from build123d import *

# Parameters (mm, degrees)
PAD_DEPTH       = 85
PAD001_DEPTH    = 6
POCKET_DEPTH    = 42.401
POCKET001_DEPTH = 48.001
FILLET_R        = 1
CHAMFER_SIZE    = 1


with BuildPart() as part:
    # Sketch → Pad (new body)
    with BuildSketch(Plane.XY):
        with BuildLine():
            Line((40, 30), (40, 0))
            ThreePointArc((0, -40), (28.284271, -28.284271), (40, 0))
            Line((0, -40), (0, -42.4))
            ThreePointArc((0, -42.4), (29.981328, -29.981328), (42.4, 0))
            Line((42.4, 48), (42.4, 0))
            Line((0, 48), (42.4, 48))
            Line((0, 48), (0, 40))
            Line((0, 40), (30, 40))
            ThreePointArc((40, 30), (37.071068, 37.071068), (30, 40))
        make_face()
    pad = extrude(amount=PAD_DEPTH)

    # Mirrored: Pad across Sketch V_Axis
    add(pad.mirror(Plane(origin=(0, 0, 0), x_dir=(0, 0, 1), z_dir=(1, 0, 0))))

    # Sketch001 → Pad001 (join)
    with BuildSketch(Plane.XY):
        Polygon((6, -41.507187), (6, -6), (40.95602, -6), (40.95602, 6), (6, 6), (6, 41.507187), (-6, 41.507187), (-6, 6), (-40.95602, 6), (-40.95602, -6), (-6, -6), (-6, -41.507187), align=None)
    extrude(amount=PAD001_DEPTH)

    # Sketch002 → Pocket (cut, through all)
    with BuildSketch(Plane.XZ):
        with BuildLine():
            Line((0, 53.283252), (-12.698919, 35.147317))
            ThreePointArc((-12.698919, 35.147317), (-13.7168, 19.617441), (-0.411638, 11.54367))
            Line((-0.411638, 11.54367), (0.411638, 11.54367))
            ThreePointArc((0.411638, 11.54367), (13.7168, 19.617441), (12.698919, 35.147317))
            Line((12.698919, 35.147317), (0, 53.283252))
        make_face()
    extrude(amount=POCKET_DEPTH, mode=Mode.SUBTRACT)

    # Sketch003 → Pocket001 (cut, through all)
    with BuildSketch(Plane.XZ):
        with BuildLine():
            ThreePointArc((27.5, 65.454356), (30, 54), (32.5, 65.454356))
            Line((32.5, 65.454356), (32.5, 75))
            ThreePointArc((32.5, 75), (30, 77.5), (27.5, 75))
            Line((27.5, 75), (27.5, 65.454356))
        make_face()
        with BuildLine():
            ThreePointArc((-32.5, 65.454356), (-30, 54), (-27.5, 65.454356))
            Line((-27.5, 65.454356), (-27.5, 75))
            ThreePointArc((-27.5, 75), (-30, 77.5), (-32.5, 75))
            Line((-32.5, 75), (-32.5, 65.454356))
        make_face()
        with BuildLine():
            ThreePointArc((-2.5, 18.617909), (0, 7.163552), (2.5, 18.617909))
            Line((2.5, 18.617909), (2.5, 28.163552))
            ThreePointArc((2.5, 28.163552), (0, 30.663552), (-2.5, 28.163552))
            Line((-2.5, 28.163552), (-2.5, 18.617909))
        make_face()
    extrude(amount=-POCKET001_DEPTH, mode=Mode.SUBTRACT)

    # Fillet
    fillet_edges = [part.edges().sort_by_distance(p)[0] for p in [
        (-40, 15, 85),
        (-28.284271, -28.284271, 85),
        (0, -41.2, 85),
        (-29.981328, -29.981328, 85),
        (-42.4, 24, 85),
        (-21.2, 48, 85),
        (0, 44, 85),
        (-15, 40, 85),
        (-37.071068, 37.071068, 85),
    ]]
    fillet(fillet_edges, radius=FILLET_R)

    # Chamfer
    chamfer_edges = [part.edges().sort_by_distance(p)[0] for p in [
        (-6, 23, 6),
        (-23, 6, 6),
        (-22.77372, -6, 6),
        (-6, -22.77372, 6),
        (6, -22.77372, 6),
        (22.77372, -6, 6),
        (23, 6, 6),
        (6, 23, 6),
    ]]
    chamfer(chamfer_edges, length=CHAMFER_SIZE)


solid = part.part
Geometry: final body of the model. Coordinates: model frame, mm. A direction names the side the tool comes from. Coordinates: 2 decimals unless noted, no trailing zeros. Order: outer loops, then holes, each group sorted by start corner. A loop starts at its lowest first (then second) coordinate and runs counter-clockwise, first axis right, second up.
(1) Section query A-A (z = 60). Return the cut outline in (x, y).
(2) Draft query along Y for faces 5 (the face through (27.5, 44, 70)), 6 (the face through (23, -6, 2)). Return one class per face: pulls with the +Y half, pulls with the -Y half, needs draft (parallel to the pull), parting line crosses it, or undercut.
(3) Section query D-D (z = 26). Return the cut outline in (x, y).
(4) Material intervals for probe 1 along X at (y, z) = (41.25, 60); probe 2 along X at (y, z) = (30, 76); probe 3 along Z at (x, y) = (0, 42), sorted ascending.
(5) First-contact query: pin 1 (7 mm diameter, centred on x = 30, z = 60, fed in from +Y); pin 2 (4 mm diameter, centred on y = -32, z = 68, fed in from +X); pin 3 (5.5 mm diameter, centred on x = -17, z = 2, fed in from -Y). Flat tips, straight axial feed; report the tip coordinate or a pass-through.
(6) Section query C-C (y = 33.5). State how many separate pieces and enclosed holes the cut face has, plus the area to 3 significant figures.
(7) Section query B-B (z = 45.5). Return the cut outline in (x, y), plus the area to 3 significant figures.
(8) Access query for faces 1 (the face through (13.6, -39, 19.4)), 2 (the face through (-27.5, 44, 70)), 3 (the face through (0.055, 43.944, 30.663)), 4 (the face through (-23, -6, 2)). Directions: +Z, -Z, +X, -X, +Y, -Y. A direction counts if a zero-diameter tool reaches every point of the face in a straight line with its end or side. Return the directions, or none.
Solution:
1. outline: (-42.4, 0) arc R42.4 ccw to (0, -42.4) arc R42.4 ccw to (42.4, 0) - (42.4, 48) - (36, 48) - (36, 38) arc R10 cw to (40, 30) - (40, 0) arc R40 cw to (0, -40) arc R40 cw to (-40, 0) - (-40, 30) arc R10 cw to (-36, 38) - (-36, 48) - (-42.4, 48) - close; (-24, 40) - (24, 40) - (24, 48) - (-24, 48) - close
2. face 5: needs draft
2. face 6: undercut
3. outline: (-42.4, 0) arc R42.4 ccw to (-15.4, -39.5) - (-15.4, -36.92) arc R40 cw to (-40, 0) - (-40, 30) arc R10 cw to (-30, 40) - (-2.5, 40) - (-2.5, 48) - (-42.4, 48) - close; (2.5, 40) - (30, 40) arc R10 cw to (40, 30) - (40, 0) arc R40 cw to (15.4, -36.92) - (15.4, -39.5) arc R42.4 ccw to (42.4, 0) - (42.4, 48) - (2.5, 48) - close
4. probe 1: x = -42.4 to -36, -24 to 24, 36 to 42.4
4. probe 2: x = -42.4 to -40, 40 to 42.4
4. probe 3: z = 0 to 7.16, 30.66 to 85
5. pin 1: stops at y = -21.86
5. pin 2: stops at x = 29.96
5. pin 3: stops at y = -39.93
6. separate pieces: 3
6. enclosed holes: 0
6. area: 586 mm2
7. outline: (-42.4, 0) arc R42.4 ccw to (-5.45, -42.05) - (-5.45, -39.63) arc R40 cw to (-40, 0) - (-40, 30) arc R10 cw to (-30, 40) - (30, 40) arc R10 cw to (40, 30) - (40, 0) arc R40 cw to (5.45, -39.63) - (5.45, -42.05) arc R42.4 ccw to (42.4, 0) - (42.4, 48) - (-42.4, 48) - close
7. area: 1,200 mm2
8. face 1: -Y
8. face 2: +Y
8. face 3: +Y, -Y
8. face 4: +Z, -Z
